```python
from build123d import *

# Parameters (mm, degrees)
SKICA1_W                 = 44
SKICA1_H                 = 108
SKICA1_W_2               = 40
SKICA1_H_2               = 104
P_IDAT_VYSUNUT_M1_DEPTH  = 25
SKICA2_W                 = 44
SKICA2_H                 = 108
P_IDAT_VYSUNUT_M2_DEPTH  = 2
ZAOBLIT1_R               = 2.5
SKICA3_W                 = 44
SKICA3_H                 = 108
SKICA3_W_2               = 42
SKICA3_H_2               = 106
ODEBRAT_VYSUNUT_M1_DEPTH = 2
SKICA4_R                 = 1.5
P_IDAT_VYSUNUT_M3_DEPTH  = 22
ODEBRAT_VYSUNUT_M2_DEPTH = 10
SKICA7_W                 = 40
SKICA7_H                 = 2
SKICA7_W_2               = 5
P_IDAT_VYSUNUT_M4_DEPTH  = 10
SKICA8_R                 = 0.95
SKICA8_W                 = 6
SKICA8_H                 = 12
ODEBRAT_VYSUNUT_M3_DEPTH = 10


with BuildPart() as part:
    # Skica1 → Přidat vysunutím1 (new body)
    with BuildSketch(Plane.XY):
        with Locations((22, 54)):
            Rectangle(SKICA1_W, SKICA1_H)
        with Locations((22, 54)):
            Rectangle(SKICA1_W_2, SKICA1_H_2, mode=Mode.SUBTRACT)
    extrude(amount=P_IDAT_VYSUNUT_M1_DEPTH)

    # Skica2 → Přidat vysunutím2 (add)
    with BuildSketch(Plane.XY.offset(25)):
        with Locations((22, 54)):
            Rectangle(SKICA2_W, SKICA2_H)
    extrude(amount=P_IDAT_VYSUNUT_M2_DEPTH)

    # Zaoblit1
    zaoblit1_edges = [part.edges().sort_by_distance(p)[0] for p in [
        (0, 108, 13.5),
        (44, 108, 13.5),
        (44, 0, 13.5),
        (0, 0, 13.5),
    ]]
    fillet(zaoblit1_edges, radius=ZAOBLIT1_R)

    # Skica3 → Odebrat vysunutím1 (cut)
    with BuildSketch(Plane(origin=(0, 0, 0), x_dir=(-1, 0, 0), z_dir=(0, 0, -1))):
        with Locations((-22, 54)):
            Rectangle(SKICA3_W, SKICA3_H)
        with Locations((-22, 54)):
            Rectangle(SKICA3_W_2, SKICA3_H_2, mode=Mode.SUBTRACT)
    extrude(amount=-ODEBRAT_VYSUNUT_M1_DEPTH, mode=Mode.SUBTRACT)

    # Skica4 → Přidat vysunutím3 (add)
    with BuildSketch(Plane(origin=(0, 0, 25), x_dir=(-1, 0, 0), z_dir=(0, 0, -1))):
        with BuildLine():
            Line((-42, 2), (-42, 10))
            ThreePointArc((-42, 10), (-36.343145751, 7.656854249), (-34, 2))
            Line((-34, 2), (-42, 2))
        make_face()
        with Locations((-39, 5)):
            Circle(SKICA4_R, mode=Mode.SUBTRACT)
        with BuildLine():
            Line((-2, 2), (-10, 2))
            ThreePointArc((-10, 2), (-7.656854249, 7.656854249), (-2, 10))
            Line((-2, 10), (-2, 2))
        make_face()
        with Locations((-5, 5)):
            Circle(SKICA4_R, mode=Mode.SUBTRACT)
        with BuildLine():
            Line((-2, 80), (-2, 76))
            Line((-2, 76), (-5, 76))
            ThreePointArc((-5, 76), (-9, 80), (-5, 84))
            Line((-5, 84), (-2, 84))
            Line((-2, 84), (-2, 80))
        make_face()
        with Locations((-5, 80)):
            Circle(SKICA4_R, mode=Mode.SUBTRACT)
        with BuildLine():
            Line((-42, 84), (-39, 84))
            ThreePointArc((-39, 84), (-35, 80), (-39, 76))
            Line((-39, 76), (-42, 76))
            Line((-42, 76), (-42, 84))
        make_face()
        with Locations((-39, 80)):
            Circle(SKICA4_R, mode=Mode.SUBTRACT)
    extrude(amount=P_IDAT_VYSUNUT_M3_DEPTH)

    # Skica6 → Odebrat vysunutím2 (cut)
    with BuildSketch(Plane.XZ):
        Polygon((22, 10.4), (15.25, 10.4), (15.25, 5), (28.75, 5), (28.75, 10.4), align=None)
    extrude(amount=-ODEBRAT_VYSUNUT_M2_DEPTH, mode=Mode.SUBTRACT)

    # Skica7 → Přidat vysunutím4 (add)
    with BuildSketch(Plane(origin=(0, 0, 25), x_dir=(-1, 0, 0), z_dir=(0, 0, -1))):
        with Locations((-22, 15)):
            Rectangle(SKICA7_W, SKICA7_H)
        with Locations((-39.5, 64.682971934)):
            Rectangle(SKICA7_W_2, SKICA7_H)
    extrude(amount=P_IDAT_VYSUNUT_M4_DEPTH)

    # Skica8 → Odebrat vysunutím3 (cut)
    with BuildSketch(Plane.ZY):
        with Locations((12.5, 35.5)):
            Circle(SKICA8_R)
        with Locations((12.5, 20.5)):
            Circle(SKICA8_R)
        with Locations((12.5, 28)):
            Rectangle(SKICA8_W, SKICA8_H)
    extrude(amount=-ODEBRAT_VYSUNUT_M3_DEPTH, mode=Mode.SUBTRACT)


solid = part.part
```
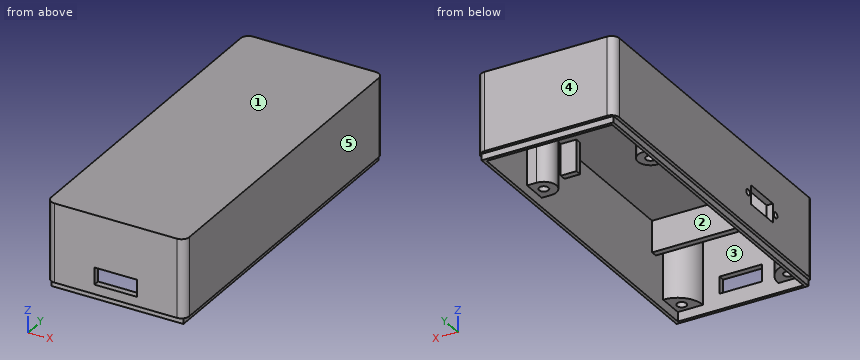
The model under review builds one solid part; all positions refer to its coordinate system, in mm. Face numbers are marked on the shaded views. A direction names the side the tool comes from. Give positions to 0.01 mm unless a question says otherwise; leave off trailing zeros. Write each loop counter-clockwise with the first axis right and the second up, starting at its lowest first coordinate (ties: lowest second). Pieces come first, ordered by that corner, then holes. Notation, with made-up numbers: (-23, 79) - (-5, 79) arc R21 cw to (-5, 105) - close; hole circle Ø8 at (-17.75, -27). An arc over 180 degrees is marked (long way). Answer in a Markdown table with one row per item. Add a question column.
1. We need section C-C on y = 25.5. Write out the cut boundary in (x, z), then the cut area to 3 significant figures.
2. We need section D-D on z = 19.5. State how many separate pieces and enclosed holes the cut face has, then the cut area to 3 significant figures.
3. Tool access review of the marked faces 1 and 2: name each direction out of +Z, -Z, +X, -X, +Y, -Y from which nothing blocks a thin tool from reaching the whole face with its end or side.
4. Wall thickness on line 1 along X through (y, z) = (80, 9.25); line 2 along X through (y, z) = (49, 9); line 3 along Y through (x, z) = (30, 13.25): over which ranges is each line inside the solid? List them lowest first. Write a range as [from, to].
5. Insertion check: P1, Ø10, axis at x = 35.5, y = 77.5, coming from the -Z side; P2, Ø4, axis at x = 4.5, y = 33.5, coming from the -Z side; P3, Ø1.6, axis at x = 19.5, y = 1.5, coming from the -Z side; P4, Ø0.6, axis at x = 1.5, z = 11.5, coming from the -Y side. Each pin has a flat end and moves straight along its axis. Give the tip position at first contact, or say it passes through.
6. Draft analysis for pull direction Y (two halves, no side actions). For the marked faces 3, 4 and 5, state which applies: +Y half, -Y half, draft (parallel to the pull), parting line (faces both ways), or undercut.
7. We need section B-B on z = 4. Write out the cut boundary in (x, y).
8. We need section A-A on x = 20.5. Write out the cut boundary in (y, z).
Ans:
| question | item | result |
|---|---|---|
| 1 | outline | (0, 2) - (1, 2) - (1, 0) - (2, 0) - (2, 9.5) - (0, 9.5) - close; (0, 15.5) - (2, 15.5) - (2, 25) - (42, 25) - (42, 0) - (43, 0) - (43, 2) - (44, 2) - (44, 27) - (0, 27) - close |
| 1 | area | 172 mm^2 |
| 2 | separate pieces | 1 |
| 2 | enclosed holes | 6 |
| 2 | area | 847 mm^2 |
| 3 | face 1 | +Z, +X, -X, +Y, -Y |
| 3 | face 2 | -Z |
| 4 | line 1 | x = [0, 3.5], [6.5, 9], [35, 37.5], [40.5, 44] |
| 4 | line 2 | x = [0, 2], [42, 44] |
| 4 | line 3 | y = [0, 2], [106, 108] |
| 5 | P1 | stops at z = 3 |
| 5 | P2 | stops at z = 25 |
| 5 | P3 | stops at z = 0 |
| 5 | P4 | stops at y = 0.1 |
| 6 | face 3 | undercut |
| 6 | face 4 | +Y half |
| 6 | face 5 | draft |
| 7 | outline | (0, 2.5) arc R2.5 ccw to (2.5, 0) - (41.5, 0) arc R2.5 ccw to (44, 2.5) - (44, 105.5) arc R2.5 ccw to (41.5, 108) - (2.5, 108) arc R2.5 ccw to (0, 105.5) - close; hole (2, 10) arc R8 cw to (10, 2) - (34, 2) arc R8 cw to (42, 10) - (42, 76) - (39, 76) arc R4 cw to (39, 84) - (42, 84) - (42, 106) - (2, 106) - (2, 84) - (5, 84) arc R4 cw to (5, 76) - (2, 76) - close; hole circle Ø3 at (5, 5); hole circle Ø3 at (5, 80); hole circle Ø3 at (39, 5); hole circle Ø3 at (39, 80) |
| 8 | outline | (0, 2) - (1, 2) - (1, 0) - (2, 0) - (2, 5) - (0, 5) - close; (0, 10.4) - (2, 10.4) - (2, 25) - (14, 25) - (14, 15) - (16, 15) - (16, 25) - (106, 25) - (106, 0) - (107, 0) - (107, 2) - (108, 2) - (108, 27) - (0, 27) - close |
